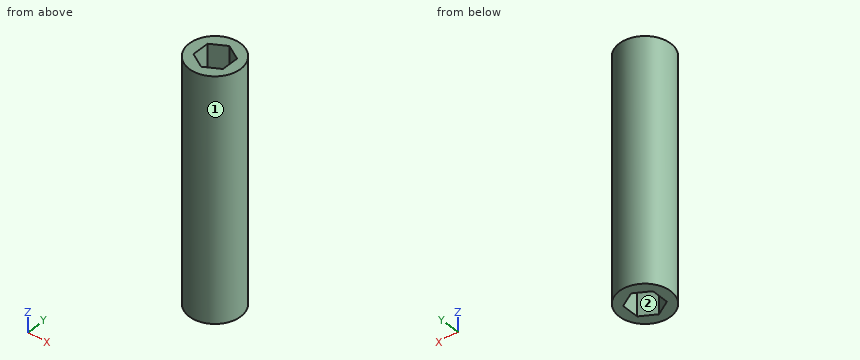
from build123d import *

# Parameters (mm, degrees)
SKETCH1_R          = 15
EXTRUDE1_DEPTH     = 141
EXTRUDE2_DEPTH     = 30
EXTRUDE3_DEPTH     = 30
SHELL5_START       = 30
SHELL5_OUTLINE_R   = 13
SHELL5_DEPTH       = 79
SHELL5_START_2     = 2
SHELL5_2_OUTLINE_R = 13
SHELL5_2_DEPTH     = 137
SHELL5_START_3     = 109
SHELL5_3_DEPTH     = 30
SHELL5_4_DEPTH     = 28
EXTRUDE4_DEPTH     = 2


# Read off the part's stored shape, not the designer's step: Shell5
with BuildPart() as part:
    # Sketch1 → Extrude1 (new body)
    with BuildSketch(Plane.XY):
        with Locations((-45.385330641, 54.653977414)):
            Circle(SKETCH1_R)
    extrude(amount=EXTRUDE1_DEPTH)

    # Sketch2 → Extrude2 (cut)
    with BuildSketch(Plane.XY.offset(141)):
        Polygon((-45.091602644, 64.656924427), (-53.813164855, 59.757219273), (-53.930676827, 49.754272261), (-45.326626587, 44.651030402), (-36.605064376, 49.550735556), (-36.487552404, 59.553682568), align=None)
    extrude(amount=-EXTRUDE2_DEPTH, mode=Mode.SUBTRACT)

    # Sketch5 → Extrude3 (cut)
    with BuildSketch(Plane(origin=(0, 0, 0), x_dir=(-1, 0, 0), z_dir=(0, 0, -1))):
        Polygon((45.385330641, 64.654606726), (36.724531603, 59.65429207), (36.724531603, 49.653662759), (45.385330641, 44.653348103), (54.046129679, 49.653662759), (54.046129679, 59.65429207), align=None)
    extrude(amount=-EXTRUDE3_DEPTH, mode=Mode.SUBTRACT)

    # Shell5 outline → Shell5 (cut)
    with BuildSketch(Plane.XY.offset(SHELL5_START)):
        with Locations((-45.385330641, 54.653977414)):
            Circle(SHELL5_OUTLINE_R)
    extrude(amount=SHELL5_DEPTH, mode=Mode.SUBTRACT)

    # Shell5 2 outline → Shell5 2 (cut)
    with BuildSketch(Plane.XY.offset(SHELL5_START_2)):
        with Locations((-45.385330641, 54.653977414)):
            Circle(SHELL5_2_OUTLINE_R)
        Polygon((-45.064474284, 66.966166161), (-34.474126219, 60.684809586), (-34.618766551, 48.37262084), (-45.353754947, 42.341788668), (-45.371174081, 42.35212032), (-45.385330641, 42.343947026), (-56.046129679, 48.49896222), (-56.046129679, 60.808992609), (-45.385330641, 66.964007803), (-45.228988272, 66.873743494), align=None, mode=Mode.SUBTRACT)
    extrude(amount=SHELL5_2_DEPTH, mode=Mode.SUBTRACT)

    # Shell5 3 outline → Shell5 3 (cut)
    with BuildSketch(Plane.XY.offset(SHELL5_START_3)):
        Polygon((-55.79946268, 60.935333989), (-45.228988272, 66.873743494), (-45.385330641, 66.964007803), (-56.046129679, 60.808992609), (-56.046129679, 48.49896222), (-45.385330641, 42.343947026), (-45.371174081, 42.35212032), (-55.944103012, 48.623145243), align=None)
    extrude(amount=SHELL5_3_DEPTH, mode=Mode.SUBTRACT)

    # Shell5 4 outline → Shell5 4 (cut)
    with BuildSketch(Plane.XY.offset(SHELL5_START_2)):
        Polygon((-34.618766551, 48.37262084), (-34.474126219, 60.684809586), (-45.064474284, 66.966166161), (-45.228988272, 66.873743494), (-34.724531603, 60.808992609), (-34.724531603, 48.49896222), (-45.371174081, 42.35212032), (-45.353754947, 42.341788668), align=None)
    extrude(amount=SHELL5_4_DEPTH, mode=Mode.SUBTRACT)

    # Sketch6 → Extrude4 (add)
    with BuildSketch(Plane.XY.offset(30)):
        Polygon((-34.724531603, 60.808992609), (-45.297222628, 66.811400248), (-55.78180564, 60.656385054), (-55.693697628, 48.49896222), (-45.121006603, 42.496554581), (-34.63642359, 48.651569775), align=None)
    extrude(amount=EXTRUDE4_DEPTH)


solid = part.part
Model file for the job. Use its own axes, mm. Face numbers are marked on the shaded views. Round coordinates to 2 decimals unless told otherwise and drop trailing zeros. Loops run counter-clockwise (first coordinate to the right, second up) from the corner with the lowest first, then second, coordinate; pieces in that order, holes last. Notation, with made-up numbers: (82.25, -18.75) -> (102.25, -18.75) arc R25 cw to (102.25, -3.75) -> close; hole circle Ø6 at (22, 15). An arc over 180 degrees is marked (long way). Answer as CSV lines item,"result". Start each with the question number.
1) Slice it at A-A (z = 13). List the corners of the cut face in (x, y).
2) Pin check, flat tips, straight feed: P1, Ø3, axis at y = 57, z = 13.5, coming from the +X side; P2, Ø12, axis at x = -43.5, y = 53.5, coming from the +Z side; P3, Ø3, axis at y = 64.5, z = 81.5, coming from the +X side. Stop position of each tip, or through.
3) Mould opens along X. For the marked faces 1 and 2 say: +X half, -X half, draft (parallel to the pull), parting line (faces both ways), or undercut.
4) Probe line 1 along Z through (x, y) = (-37.25, 48.75); line 2 along Y through (x, z) = (-47, 18.5); line 3 along Y through (x, z) = (-53, 133.5). List the from-to ranges inside material, lowest first.
5) Slice it at D-D (z = 115.5). List the corners of the cut face in (x, y).
Filled in:
1,outline,"circle Ø30 at (-45.39, 54.65); (-56.05, 48.5) -> (-45.39, 42.34) -> (-34.72, 48.5) -> (-34.72, 60.81) -> (-45.39, 66.96) -> (-56.05, 60.81) -> close; hole circle Ø26 at (-45.39, 54.65); hole (-54.05, 49.65) -> (-45.39, 44.65) -> (-36.72, 49.65) -> (-36.72, 59.65) -> (-45.39, 64.65) -> (-54.05, 59.65) -> close"
2,P1,"stops at x = -30.41"
2,P2,"stops at z = 111"
2,P3,"stops at x = -32.92"
3,face 1,"parting line"
3,face 2,"undercut"
4,line 1,"z = 0 to 32, 109 to 141"
4,line 2,"y = 39.74 to 41.75, 43.28 to 45.59, 63.72 to 66.03, 67.55 to 69.57"
4,line 3,"y = 41.73 to 44.12, 46.88 to 49.2, 60.21 to 62.51, 65.19 to 67.58"
5,outline,"circle Ø30 at (-45.39, 54.65); (-55.94, 48.62) -> (-45.35, 42.34) -> (-34.62, 48.37) -> (-34.47, 60.68) -> (-45.06, 66.97) -> (-55.8, 60.94) -> close; hole circle Ø26 at (-45.39, 54.65); hole (-53.93, 49.75) -> (-45.33, 44.65) -> (-36.61, 49.55) -> (-36.49, 59.55) -> (-45.09, 64.66) -> (-53.81, 59.76) -> close"
